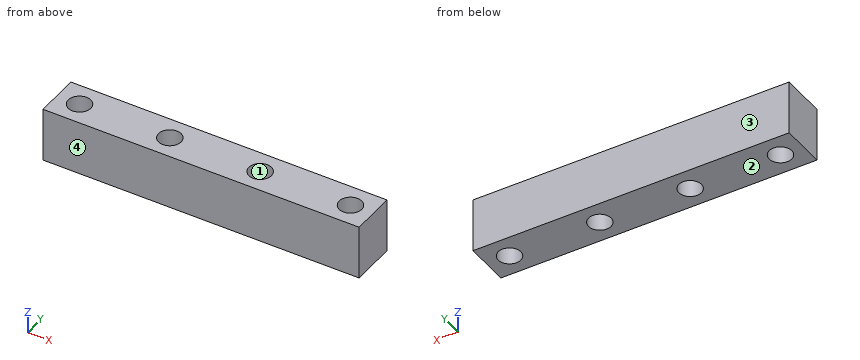
```python
from build123d import *

# Parameters (mm, degrees)
SKETCH2_W           = 44.45
SKETCH2_H           = 6.35
BOSS_EXTRUDE1_DEPTH = 7.62
SKETCH4_R           = 1.5875
CUT_EXTRUDE2_DEPTH  = 8.62


with BuildPart() as part:
    # Sketch2 → Boss-Extrude1 (new body)
    with BuildSketch(Plane.XY):
        Rectangle(SKETCH2_W, SKETCH2_H)
    extrude(amount=BOSS_EXTRUDE1_DEPTH)

    # Sketch4 → Cut-Extrude2 (cut, through all)
    with BuildSketch(Plane(origin=(0, 0, 0), x_dir=(-1, 0, 0), z_dir=(0, 0, -1))):
        with Locations((-6.35, 0)):
            Circle(SKETCH4_R)
        with Locations((-19.05, 0)):
            Circle(SKETCH4_R)
    cut_extrude2 = extrude(amount=-CUT_EXTRUDE2_DEPTH, mode=Mode.SUBTRACT)

    # Mirror2: Cut-Extrude2 across plane
    add(cut_extrude2.mirror(Plane(origin=(0, 0, 0), x_dir=(0, 0, 1), z_dir=(1, 0, 0))), mode=Mode.SUBTRACT)


solid = part.part
```
Source: CAD feature listing. Evaluate the final solid. Frame: model axes, mm. Face numbers are marked on the shaded views. Coordinates: 2 decimals unless noted, no trailing zeros. Write each loop counter-clockwise with the first axis right and the second up, starting at its lowest first coordinate (ties: lowest second). Pieces come first, ordered by that corner, then holes. Notation, with made-up numbers: (56.25, 11.5) -> (107.25, 11.5) arc R16 ccw to (107.25, 39.5) -> close; hole circle Ø10 at (-1, 87). An arc over 180 degrees is marked (long way). Return JSON: item names as keys, results as strings. Group by question number.
1) Section query B-B, the plane z = 2.5. State how many separate pieces and enclosed holes the cut face has, plus the area to 3 significant figures.
2) Section query D-D, the plane x = -6. Return loops of the section in (y, z) (3 decimals), plus the area to 3 significant figures.
3) Ray query, line 1 along X through (y, z) = (-0.75, 4.25) (3 decimals); line 2 along X through (y, z) = (-1, 4.5) (3 decimals); line 3 along Y through (x, z) = (-19.05, 5.25) (1 decimal). Return the intervals inside material, ascending.
4) Mould query, pull axis Y, two halves, no side actions, for the marked faces 1, 2, 3 and 4. Classes: +Y half, -Y half, draft (parallel to the pull), parting line (faces both ways), or undercut.
5) Section query C-C, the plane y = -0.75. Return loops of the section in (x, z) (3 decimals).
6) Section query A-A, the plane x = 19.05. Return loops of the section in (y, z) (1 decimal), plus the area to 3 significant figures.
From the geometry:
{
 "1": {"separate pieces": "1", "enclosed holes": "4", "area": "251 mm²"},
 "2": {"outline": "(-3.175, 0) -> (-1.548, 0) -> (-1.548, 7.62) -> (-3.175, 7.62) -> close; (1.548, 0) -> (3.175, 0) -> (3.175, 7.62) -> (1.548, 7.62) -> close", "area": "24.8 mm²"},
 "3": {"line 1": "-22.225 to -20.449, -17.651 to -7.749, -4.951 to 4.951, 7.749 to 17.651, 20.449 to 22.225", "line 2": "-22.225 to -20.283, -17.817 to -7.583, -5.117 to 5.117, 7.583 to 17.817, 20.283 to 22.225", "line 3": "-3.2 to -1.6, 1.6 to 3.2"},
 "4": {"face 1": "undercut", "face 2": "draft", "face 3": "+Y half", "face 4": "-Y half"},
 "5": {"outline": "(-22.225, 0) -> (-20.449, 0) -> (-20.449, 7.62) -> (-22.225, 7.62) -> close; (-17.651, 0) -> (-7.749, 0) -> (-7.749, 7.62) -> (-17.651, 7.62) -> close; (-4.951, 0) -> (4.951, 0) -> (4.951, 7.62) -> (-4.951, 7.62) -> close; (7.749, 0) -> (17.651, 0) -> (17.651, 7.62) -> (7.749, 7.62) -> close; (20.449, 0) -> (22.225, 0) -> (22.225, 7.62) -> (20.449, 7.62) -> close"},
 "6": {"outline": "(-3.2, 0) -> (-1.6, 0) -> (-1.6, 7.6) -> (-3.2, 7.6) -> close; (1.6, 0) -> (3.2, 0) -> (3.2, 7.6) -> (1.6, 7.6) -> close", "area": "24.2 mm²"}
}
